from build123d import *

# Parameters (mm, degrees)
SKETCH1_R           = 3
BOSS_EXTRUDE1_DEPTH = 6
BOSS_EXTRUDE2_DEPTH = 7
SKETCH3_R           = 3.5
BOSS_EXTRUDE3_DEPTH = 1
SKETCH4_W           = 10
SKETCH4_H           = 12
BOSS_EXTRUDE4_DEPTH = 7
SKETCH5_R           = 1.1
BOSS_EXTRUDE5_DEPTH = 4
SKETCH6_R           = 0.6
BOSS_EXTRUDE6_DEPTH = 4


with BuildPart() as part:
    # Sketch1 → Boss-Extrude1 (new body)
    with BuildSketch(Plane(origin=(0, 0, 0), x_dir=(1, 0, 0), z_dir=(0, 1, 0))):
        with Locations(Location((0, 1, 0), (0, 0, 270))):
            Circle(SKETCH1_R)
    extrude(amount=BOSS_EXTRUDE1_DEPTH)

    # Sketch2 → Boss-Extrude2 (add)
    with BuildSketch(Plane(origin=(0, 6, 0), x_dir=(1, 0, 0), z_dir=(0, 1, 0))):
        with BuildLine():
            Line((-2.653299832, -0.4), (2.653299832, -0.4))
            ThreePointArc((2.653299832, -0.4), (0, 4), (-2.653299832, -0.4))
        make_face()
    extrude(amount=BOSS_EXTRUDE2_DEPTH)

    # Sketch3 → Boss-Extrude3 (add)
    with BuildSketch(Plane.XZ):
        with Locations(Location((0, -1, 0), (0, 0, 270))):
            Circle(SKETCH3_R)
    extrude(amount=BOSS_EXTRUDE3_DEPTH)

    # Sketch4 → Boss-Extrude4 (add)
    with BuildSketch(Plane.XZ.offset(1)):
        Rectangle(SKETCH4_W, SKETCH4_H)
    extrude(amount=BOSS_EXTRUDE4_DEPTH)

    # Sketch5 → Boss-Extrude5 (add)
    with BuildSketch(Plane.XZ.offset(8)):
        with Locations(Location((-5.001245267, 0, 0), (0, 0, 89.93513768))):
            Circle(SKETCH5_R)
        with Locations(Location((5, 0, 0), (0, 0, 270))):
            Circle(SKETCH5_R)
    extrude(amount=BOSS_EXTRUDE5_DEPTH)

    # Sketch6 → Boss-Extrude6 (add)
    with BuildSketch(Plane.XZ.offset(8)):
        with Locations(Location((0, 6, 0), (0, 0, 180))):
            Circle(SKETCH6_R)
        with Locations(Location((2.5, 6, 0), (0, 0, 180))):
            Circle(SKETCH6_R)
        with Locations(Location((-2.5, 6, 0), (0, 0, 180))):
            Circle(SKETCH6_R)
    extrude(amount=BOSS_EXTRUDE6_DEPTH)


solid = part.part
For this review, take the finished solid that the model builds, in its own axes (mm). A direction names the side the tool comes from. Round coordinates to 2 decimals unless told otherwise and drop trailing zeros. Loops run counter-clockwise (first coordinate to the right, second up) from the corner with the lowest first, then second, coordinate; pieces in that order, holes last. Notation, with made-up numbers: (-3.75, 61) - (19.25, 61) arc R16 cw to (19.25, 71) - close; hole circle Ø9 at (43, 54). An arc over 180 degrees is marked (long way). One line per item, written item: value. Start each with the question number.
Item 1: Clearance check with flat-ended pins moving along their axes: pin 1 Ø0.9 at (x, z) = (-6, -0.5) entering from +Y; pin 2 Ø0.7 at (x, z) = (-2.5, 6) entering from +Y; pin 3 Ø6 at (x, y) = (0, 9.5) entering from +Z. State where each tip first meets the part, or that it passes through.
Item 2: Take a section at A-A (y = -7.75). Give the boundary of the cut face in (x, z).
Item 3: The part is to be moulded in two halves that separate along X. For faces 5 (the flat face through (-2.5, -12, 6)), 6 (the flat face through (0, -8, 0)), 7 (the flat face through (-5, -4, 0)), say which applies: +X half, -X half, draft (parallel to the pull), parting line (faces both ways), or undercut.
Item 4: Take a section at D-D (y = 9.5). Give the boundary of the cut face in (x, z).
Item 5: For L1, parallel to Y at x = 0.5, z = -4.75; L2, parallel to X at y = -5.5, z = -2; L3, parallel to Z at x = -0.25, y = -3, list the stretches that pass through material, from the lowest coordinate up.
Item 6: Take a section at B-B (z = 2.25). Give the boundary of the cut face in (x, y), plus the area to 3 significant figures.
Item 7: Take a section at C-C (z = 5.75). Give the boundary of the cut face in (x, y).
Item 8: For faces 1 (the flat face through (5.4, -8, 0)), 2 (the cylindrical face through (-3.928, -9.972, -0.24)), 3 (the flat face through (0, -4, 6)), 4 (the flat face through (-5.4, -8, 0)), list the 3-axis set-ups (+Z, -Z, +X, -X, +Y, -Y) from which the entire face can be reached by the end or side of a thin tool; tool diameter is ignored.
Answer below:
1. pin 1: stops at y = -8
1. pin 2: stops at y = -1
1. pin 3: stops at z = 0.4
2. outline: (-5, -6) - (5, -6) - (5, 6) - (-5, 6) - close
3. face 5: draft
3. face 6: undercut
3. face 7: -X half
4. outline: (-2.65, 0.4) arc R3 ccw (long way) to (2.65, 0.4) - close
5. L1: y = -8 to -1
5. L2: x = -5 to 5
5. L3: z = -6 to 6
6. outline: (-5, -8) - (5, -8) - (5, -1) - (1.3, -1) - (1.3, 0) - (-1.3, 0) - (-1.3, -1) - (-5, -1) - close
6. area: 72.6 mm2
7. outline: (-5, -8) - (-3.05, -8) - (-3.05, -12) - (-1.95, -12) - (-1.95, -8) - (-0.55, -8) - (-0.55, -12) - (0.55, -12) - (0.55, -8) - (1.95, -8) - (1.95, -12) - (3.05, -12) - (3.05, -8) - (5, -8) - (5, -1) - (-5, -1) - close
8. face 1: +Z, -Z, +X, +Y
8. face 2: -Y
8. face 3: +Z, +X, -X, +Y
8. face 4: +Z, -Z, -X, +Y
